from build123d import *

# Parameters (mm, degrees)
BASPROSKE_W        = 12
BASPROSKE_H        = 20.25
TOOTHCUT_DEPTH     = 32.050362317
TEETHCUTS_COUNT    = 25
TEETHCUTS_ANGLE    = 345.6
HUBNEABOTSKE_R     = 7.5
HUBNEARBOTH_DEPTH  = 7.7500254
HUBFAR_START       = 7.7500254
HUBFARSKE_R        = 7.5
HUBFAR_DEPTH       = 7.7500254
BORSKE_R           = 3
BORE_DEPTH         = 27.5000508
SKETCH1_R          = 2
CUT_EXTRUDE1_DEPTH = 15


with BuildPart() as part:
    # BasProSke → Base-Revolve (revolve)
    with BuildSketch(Plane(origin=(0, 0, 0), x_dir=(1, 0, 0), z_dir=(0, 1, 0)), mode=Mode.PRIVATE) as base_revolve_sk:
        with Locations((6, 10.125)):
            Rectangle(BASPROSKE_W, BASPROSKE_H)
    revolve(base_revolve_sk.sketch.rotate(Axis((-10, 0, 0), (1, 0, 0)), 180), axis=Axis((-10, 0, 0), (1, 0, 0)))

    # TooCutSke → ToothCut (cut, through all)
    with BuildSketch(Plane(origin=(0, 0, 0), x_dir=(0, 0, -1), z_dir=(1, 0, 0))):
        with BuildLine():
            ThreePointArc((0.713909619, 16.858891098), (0, 16.874), (-0.713909619, 16.858891098))
            ThreePointArc((-0.713909619, 16.858891098), (-1.221902209, 18.597177626), (-2.131751691, 20.163022588))
            ThreePointArc((-2.131751691, 20.163022588), (0, 20.2754), (2.131751691, 20.163022588))
            ThreePointArc((2.131751691, 20.163022588), (1.221902209, 18.597177626), (0.713909619, 16.858891098))
        make_face()
    toothcut = extrude(amount=TOOTHCUT_DEPTH, mode=Mode.SUBTRACT)

    # TeethCuts: ToothCut ×25 about axis
    teethcuts_axis = Axis((-10, 0, 0), (1, 0, 0))
    for i in range(1, TEETHCUTS_COUNT):
        add(toothcut.rotate(teethcuts_axis, i * TEETHCUTS_ANGLE / (TEETHCUTS_COUNT - 1)), mode=Mode.SUBTRACT)

    # HubNeaBotSke → HubNearBoth (add)
    with BuildSketch(Plane.ZY):
        with Locations(Location((0, 0, 0), (0, 0, 180))):
            Circle(HUBNEABOTSKE_R)
    extrude(amount=HUBNEARBOTH_DEPTH)

    # HubFarSke → HubFar (add)
    with BuildSketch(Plane(origin=(12, 0, 0), x_dir=(0, 0, -1), z_dir=(1, 0, 0)).offset(HUBFAR_START)):
        Circle(HUBFARSKE_R)
    extrude(amount=-HUBFAR_DEPTH)

    # BorSke → Bore (cut, symmetric)
    with BuildSketch(Plane(origin=(0, 0, 0), x_dir=(0, 0, -1), z_dir=(1, 0, 0))):
        with Locations(Location((0, 0, 0), (0, 0, 180))):
            Circle(BORSKE_R)
    extrude(amount=BORE_DEPTH, both=True, mode=Mode.SUBTRACT)

    # Sketch1 → Cut-Extrude1 (cut)
    with BuildSketch(Plane.ZY):
        with Locations((-8.700018149, -7.520617276)):
            Circle(SKETCH1_R)
    extrude(amount=-CUT_EXTRUDE1_DEPTH, mode=Mode.SUBTRACT)


solid = part.part
The listing builds one solid part. Answer for the finished solid, in the listing's coordinates (mm). A direction names the side the tool comes from. Round coordinates to 2 decimals unless told otherwise and drop trailing zeros. Order: outer loops, then holes, each group sorted by start corner. A loop starts at its lowest first (then second) coordinate and runs counter-clockwise, first axis right, second up. Notation, with made-up numbers: M 27,-0.5 L 69,-0.5 A22 cw 69,11.5 Z; hole C 1,88.5 d10. An arc over 180 degrees is marked long. Answer in a Markdown table with one row per item. Add a question column.
1) The part is cut by section A-A on x = 16.75. Determine the outline of the cut face in (y, z), plus the area to 3 significant figures.
2) The part is cut by section B-B on x = 9. Count the separate pieces of the cut face and the enclosed holes in it, plus the area to 3 significant figures.
3) Determine the mould class of faces 6 (the face through (5.92, 2.39, 18.49)), 7 (the face through (0, -9, 0)), 8 (the face through (5.916, -14.333, 11.929)) for opening direction Z: pulls with the +Z half, pulls with the -Z half, needs draft (parallel to the pull), parting line crosses it, or undercut.
4) Consider line 1 along Y through (x, z) = (1, 0); line 2 along Z through (x, y) = (6, -14); line 3 along Z through (x, y) = (8.5, 18). Determine where each line is inside the solid, lowest interval first. Write a range as from..to.
5) Which of the six approach directions +Z, -Z, +X, -X, +Y, -Y give full straight-line access (tool end or side, diameter ignored) to faces 1 (the face through (5.916, 15.715, -10.038)), 2 (the face through (5.916, 8.935, -16.367)), 3 (the face through (-7.75, -0.1, -3.2)), 4 (the face through (5.916, 11.005, 15.053)), 5 (the face through (5.916, -0.055, -18.647))?
6) Flat-ended cylindrical pins translate along their axes: pin 1 Ø12 at (y, z) = (-14, -16) entering from -X; pin 2 Ø12 at (x, y) = (10, -16) entering from -Z; pin 3 Ø9.5 at (y, z) = (0, 0) entering from -X; pin 4 Ø10 at (x, y) = (9, 6) entering from +Z. Find the tip coordinate at first contact, or state that the pin passes through.
Findings below:
| question | item | result |
|---|---|---|
| 1 | outline | C 0,0 d15; hole C 0,0 d6 |
| 1 | area | 148 mm² |
| 2 | separate pieces | 1 |
| 2 | enclosed holes | 2 |
| 2 | area | 1,030 mm² |
| 3 | face 6 | pulls with the +Z half |
| 3 | face 7 | needs draft |
| 3 | face 8 | undercut |
| 4 | line 1 | y = -20.25..-3, 3..16.87 |
| 4 | line 2 | z = -14.04..-11.42, -9.42..9.42, 11.42..14.04 |
| 4 | line 3 | z = -7.91..-6.04, -3.48..-1, 1..3.48, 6.04..7.91 |
| 5 | face 1 | +X, -X, +Y |
| 5 | face 2 | +X, -X |
| 5 | face 3 | +Z, -Z, -X, +Y, -Y |
| 5 | face 4 | +Z, +X, -X |
| 5 | face 5 | -Z, +X, -X |
| 6 | pin 1 | stops at x = 0 |
| 6 | pin 2 | stops at z = -17.32 |
| 6 | pin 3 | stops at x = -7.75 |
| 6 | pin 4 | stops at z = 19.97 |
